from build123d import *

# Parameters (mm, degrees)
BOSS_EXTRUDE1_DEPTH = 304.8
SKETCH2_W           = 30
SKETCH2_H           = 30
BOSS_EXTRUDE2_DEPTH = 2.5
SKETCH3_R           = 4
CUT_EXTRUDE1_DEPTH  = 311.214909377


with BuildPart() as part:
    # Sketch1 → Boss-Extrude1 (new body)
    with BuildSketch(Plane.XY):
        Polygon((0, 0), (0, 30), (2.5, 30), (2.5, 2.5), (30, 2.5), (30, 0), align=None)
    extrude(amount=BOSS_EXTRUDE1_DEPTH)

    # Sketch2 → Boss-Extrude2 (add)
    with BuildSketch(Plane(origin=(0, 0, 0), x_dir=(-1, 0, 0), z_dir=(0, 0, -1))):
        with Locations((-15, 15)):
            Rectangle(SKETCH2_W, SKETCH2_H)
    extrude(amount=BOSS_EXTRUDE2_DEPTH)

    # Sketch3 → Cut-Extrude1 (cut, through all)
    with BuildSketch(Plane(origin=(0, 0, -2.5), x_dir=(-1, 0, 0), z_dir=(0, 0, -1))):
        with Locations((-15, 15)):
            Circle(SKETCH3_R)
    extrude(amount=-CUT_EXTRUDE1_DEPTH, mode=Mode.SUBTRACT)


solid = part.part
Design review of the part built by this model. Coordinates are the model's own, in mm. A direction names the side the tool comes from. Round coordinates to 2 decimals unless told otherwise and drop trailing zeros. Loops run counter-clockwise (first coordinate to the right, second up) from the corner with the lowest first, then second, coordinate; pieces in that order, holes last. Notation, with made-up numbers: (23, 17) - (68, 17) arc R7 ccw to (68, 28) - close; hole circle Ø3 at (-2.75, 62). An arc over 180 degrees is marked (long way). One line per item, written item: value. Start each with the question number.
1) To check wall thickness, follow L1, parallel to Y at x = 15, z = -1.3; L2, parallel to Y at x = 29.25, z = 126; L3, parallel to Z at x = 4.75, y = 11.5. State the ranges of each line that lie inside material, in increasing order. Write a range as from..to.
2) Consider section C-C on z = 192.5. Give the boundary of the cut face in (x, y), then the cut area to 3 significant figures.
3) For faces 4 (the flat face through (16.4, 19.5, 0)), 5 (the flat face through (19, 12, -2.5)), list the 3-axis set-ups (+Z, -Z, +X, -X, +Y, -Y) from which the entire face can be reached by the end or side of a thin tool; tool diameter is ignored.
4) Consider section A-A on y = 15. Give the boundary of the cut face in (x, z).
5) Draft analysis for pull direction Y (two halves, no side actions). For faces 1 (the cylindrical face through (17.95, 17.7, -1.27)), 2 (the flat face through (1, 30, 152)), 3 (the flat face through (2.5, 16, 150)), state which applies: +Y half, -Y half, draft (parallel to the pull), parting line (faces both ways), or undercut.
6) Insertion check: pin 1 Ø3 at (x, z) = (9.5, 81.5) entering from +Y; pin 2 Ø14 at (x, y) = (12.5, 21) entering from +Z; pin 3 Ø12 at (y, z) = (3.5, 126) entering from -X; pin 4 Ø8 at (y, z) = (13.5, 154.5) entering from +X. Each pin has a flat end and moves straight along its axis. Give the tip position at first contact, or say it passes through.
Reported:
1. L1: y = 0..11, 19..30
1. L2: y = 0..2.5
1. L3: z = -2.5..0
2. outline: (0, 0) - (30, 0) - (30, 2.5) - (2.5, 2.5) - (2.5, 30) - (0, 30) - close
2. area: 144 mm^2
3. face 4: +Z, +X, +Y
3. face 5: -Z, +X, -X, +Y, -Y
4. outline: (0, -2.5) - (11, -2.5) - (11, 0) - (2.5, 0) - (2.5, 304.8) - (0, 304.8) - close; (19, -2.5) - (30, -2.5) - (30, 0) - (19, 0) - close
5. face 1: undercut
5. face 2: +Y half
5. face 3: draft
6. pin 1: stops at y = 2.5
6. pin 2: stops at z = 0
6. pin 3: stops at x = 0
6. pin 4: stops at x = 2.5
